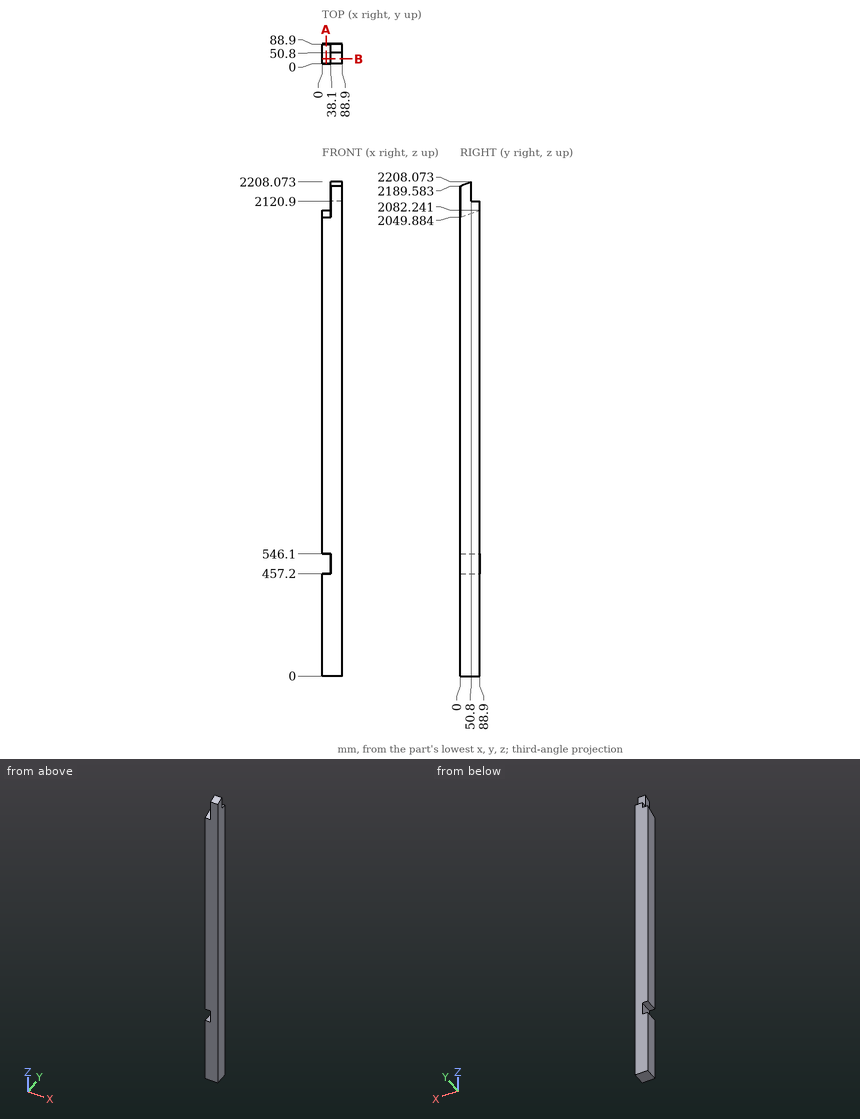
Part print with two shaded views. Sizes in mm from the minimum x, y, z corner. Coordinates: 2 decimals unless noted, no trailing zeros. Order: outer loops, then holes, each group sorted by start corner. A loop starts at its lowest first (then second) coordinate and runs counter-clockwise, first axis right, second up. Notation, with made-up numbers: (-21.75, -7) - (5.25, -7) arc R17 cw to (5.25, 2) - close; hole circle Ø5 at (54, -12.5). An arc over 180 degrees is marked (long way). Write item = value, one per line. Start each with the question number.
1) Saw through at A-A on x = 18. Write the cut outline in (y, z).
2) Flat gauge pins, fed straight in: pin 1 Ø19 at (x, y) = (27.5, 66) entering from +Z; pin 2 Ø11.5 at (x, y) = (15.5, 64) entering from -Z. Where does each tip first touch, or does it go through?
3) Saw through at B-B on y = 22. Write the cut outline in (x, z).
4) Wall check: line 1 along Z through (x, y) = (78.5, 70); line 2 along Z through (x, y) = (30.5, 10.5); line 3 along Z through (x, y) = (28.5, 42). Give the ranges that are in metal, low to high. Write a range as from..to.
From the geometry:
q1.outline = (0, 0) - (88.9, 0) - (88.9, 457.2) - (0, 457.2) - close; (0, 546.1) - (88.9, 546.1) - (88.9, 2082.24) - (0, 2049.88) - close
q2.pin_1 = 2077.36
q2.pin_2 = 0
q3.outline = (0, 0) - (88.9, 0) - (88.9, 2197.59) - (38.1, 2197.59) - (38.1, 2057.89) - (0, 2057.89) - (0, 546.1) - (38.1, 546.1) - (38.1, 457.2) - (0, 457.2) - close
q4.line_1 = 0..2120.9
q4.line_2 = 0..457.2, 546.1..2053.71
q4.line_3 = 0..457.2, 546.1..2065.17
